Input: part model. Units: mm. Frame: model coordinates. Face numbers are marked on the shaded views. A direction names the side the tool comes from. Round coordinates to 2 decimals unless told otherwise and drop trailing zeros. Loops run counter-clockwise (first coordinate to the right, second up) from the corner with the lowest first, then second, coordinate; pieces in that order, holes last. Notation, with made-up numbers: (24.25, 42.5) - (56.25, 42.5) arc R12 ccw to (56.25, 62.5) - close; hole circle Ø2 at (19.5, -33.75). An arc over 180 degrees is marked (long way). Write each question's results on one line, items separated by ' | '.
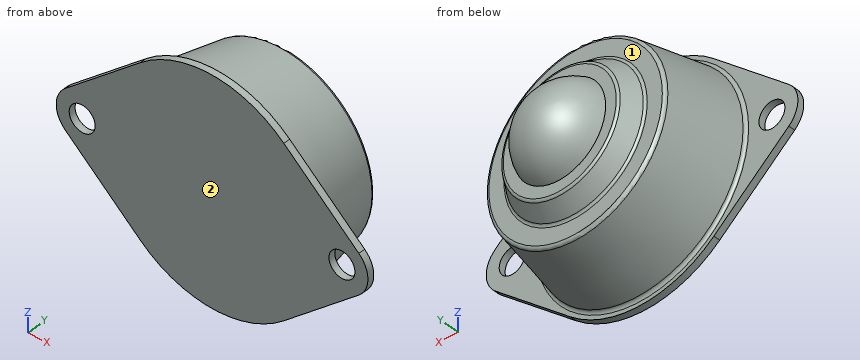
Autodesk Inventor part; units mm, degrees
ref_plane "YZ Plane" through (0, 0, 0) normal (1, 0, 0) x (0, 1, 0)
ref_plane "XZ Plane" through (0, 0, 0) normal (0, 1, 0) x (-1, 0, 0)
ref_plane "XY Plane" through (0, 0, 0) normal (0, 0, 1) x (1, 0, 0)
sketch "Skizze2" plane through (0, 0, 0) normal (0, 0, 1) x (1, 0, 0)
  line L0 (-7.07, 14) -> (-8.97, 14)
  line L1 (-8.97, 14) -> (-10.77, 11.3)
  line L2 (-10.77, 11.3) -> (-13.77, 11.3)
  line L3 (-13.77, 11.3) -> (-16, 0)
  line L4 (-16, 0) -> (-15, 0)
  line L5 (-15, 0) -> (-12.9673, 10.3)
  line L6 (-12.9673, 10.3) -> (-10.2348, 10.3)
  line L7 (-10.2348, 10.3) -> (-9.3538, 11.6215)
  line L8 (0, -2.8203) -> (0, 16.9217)
  line L9 (-6.4694, 0) -> (0, 0)
  line L10 (0, 0) -> (0, 4)
  line L11 (0, 4) -> (-6.4694, 4)
  line L12 (-6.4694, 4) -> (-6.4694, 0)
  arc A0 (-7.07, 14) -> (-9.3538, 11.6215) centre (-1.5666, 6.43) ccw
  point P0 (-15.5, 0)
  point P1 (-3.2347, 0)
  dimension "d1" = 14
  dimension "d2" = 1.9
  dimension "d5" = 1.8
  dimension "d8" = 1
  dimension "d9" = 1
  dimension "d10" = 1
  dimension "d15" = 2.7
  dimension "d52" = 7.07
  dimension "d53" = 10
  dimension "d54" = 6.4694
  dimension "d58" = 9.3591
  dimension "d60" = 16
  dimension "d61" = 3
revolve "Umdrehung1" add sketch "Skizze2" angle 360 about axis through (0, -10, 0) along (0, 1, 0)
sketch "Skizze3" plane through (0, 0, 0) normal (0, 1, 0) x (-1, 0, 0)
  circle A0 centre (20, 0) radius 2
  circle A1 centre (-20, 0) radius 2
  circle A2 centre (0, 0) radius 16 construction
  arc A3 (22.6, -3.0397) -> (22.6, 3.0397) centre (20, 0) ccw
  arc A4 (-22.6, 3.0397) -> (-22.6, -3.0397) centre (-20, 0) ccw
  line L0 (22.6, -3.0397) -> (11.05, -12.9189)
  line L1 (22.6, -3.0397) -> (22.6, 13.4844) construction
  line L2 (22.6, 3.0397) -> (11.05, 12.9189)
  line L3 (-11.05, 12.9189) -> (-22.6, 3.0397)
  line L4 (-22.6, -3.0397) -> (-11.05, -12.9189)
  arc A5 (11.05, 12.9189) -> (-11.05, 12.9189) centre (0, 0) ccw
  arc A6 (-11.05, -12.9189) -> (11.05, -12.9189) centre (0, 0) ccw
  line L5 (0, -19.9813) -> (0, 17.4256) construction
  circle A7 centre (0, 0) radius 17 construction
  point P0 (0, -17)
  point P1 (0, 17)
  dimension "d32" = 36
  dimension "d33" = 40
  dimension "d34" = 20
  dimension "d36" = 4
  dimension "d37" = 8
  dimension "d38" = 8
  dimension "d39" = 4
  dimension "d42" = 1
extrude "Extrusion1" add sketch "Skizze3" against normal blind 1
sketch "Skizze4" plane through (0, 0, 0) normal (0, 0, 1) x (1, 0, 0)
  arc A0 (0, 19) -> (0, 4) centre (0, 11.5) ccw
  line L0 (7.07, 14) -> (-7.07, 14)
  line L1 (0, 4) -> (-20.7674, 4) construction
  line L2 (0, 19) -> (0, 4)
  point P0 (0, 0)
  point P1 (0, 11.5)
  dimension "d45" = 15
  dimension "d46" = 5
revolve "Umdrehung2" add sketch "Skizze4" angle 360 about axis through (0, 19, 0) along (0, -1, 0)
fillet "Rundung1" radius 0.5 4 edges at (8.97, 14, 0) (10.77, 11.3, 0) (13.77, 11.3, 0) (16, 0, 0)
properties part number "MetallKugellager_V1"
1. Line query: line 1 (Y direction, x = 8.5, z = 9.5); line 2 (Y direction, x = -6, z = 9); line 3 (Z direction, x = -20, y = -0.45). Output: solid intervals per line, ascending. Write a range as [from, to].
Answer:
line 1: [-1, 0], [10.3, 11.3] | line 2: [-1, 0], [10.3, 11.35] | line 3: [-5.26, -2], [2, 5.26]
2. Section query B-B, the plane y = 8.25. Output: boundary loops of the cut face in (x, z), plus the area to 3 significant figures.
Answer:
outline: circle Ø28.74 at (0, 0); circle Ø13.52 at (0, 0); hole circle Ø26.74 at (0, 0) | area: 231 mm^2
3. Section query C-C, the plane y = 1.25. Output: boundary loops of the cut face in (x, z), plus the area to 3 significant figures.
Answer:
outline: circle Ø31.51 at (0, 0); circle Ø12.94 at (0, 0); hole circle Ø29.51 at (0, 0) | area: 227 mm^2
4. Section query A-A, the plane x = 19. Output: boundary loops of the cut face in (y, z), plus the area to 3 significant figures.
Answer:
outline: (-1, -6.12) - (0, -6.12) - (0, -1.73) - (-1, -1.73) - close; (-1, 1.73) - (0, 1.73) - (0, 6.12) - (-1, 6.12) - close | area: 8.77 mm^2
5. Set-up query: the marked faces 1 and 2. Return all of +Z, -Z, +X, -X, +Y, -Y with unobstructed straight access to the full face (end or side cutting, diameter ignored); none if empty.
Answer:
face 1: +Y | face 2: +Z, -Z, +X, -X, -Y
6. Contact query for flat-ended pins moving along their axis: pin 1 (8 mm diameter, centred on x = -10, y = 15.5, fed in from -Z); pin 2 (3 mm diameter, centred on x = 20, z = 0, fed in from -Y); pin 3 (5 mm diameter, centred on y = 8, z = 11.5, fed in from -X); pin 4 (10 mm diameter, centred on x = -11.5, z = 4.5, fed in from +Y). Output: stop coordinate, or through.
Answer:
pin 1: z = -6.77 | pin 2: through | pin 3: x = -11.37 | pin 4: y = 14
